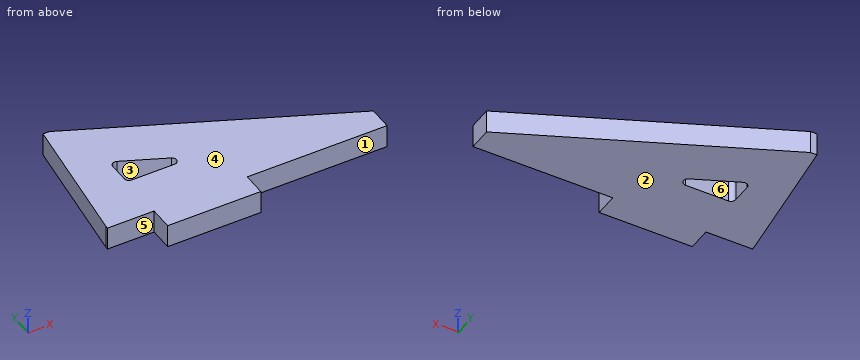
```python
from build123d import *

# Parameters (mm, degrees)
BOSS_EXTRUDE1_DEPTH = 6.35
CUT_EXTRUDE1_DEPTH  = 78.771299333


with BuildPart() as part:
    # Sketch2 → Boss-Extrude1 (new body)
    with BuildSketch(Plane.XY):
        Polygon((0, 0), (0, 6.35), (-12.7, 6.35), (-12.7, 44.45), (-6.35, 44.45), (63.5, 12.7), (63.5, 6.35), (25.4, 6.35), (25.4, 0), align=None)
        with BuildLine():
            Line((0, 25.64089525), (0, 20.32))
            ThreePointArc((0, 20.32), (0.371974388, 19.421974388), (1.27, 19.05))
            Line((1.27, 19.05), (12.97596955, 19.05))
            ThreePointArc((12.97596955, 19.05), (14.217184699, 20.051141386), (13.501499289, 21.476165426))
            Line((13.501499289, 21.476165426), (1.795529739, 26.797060676))
            ThreePointArc((1.795529739, 26.797060676), (0.5824401, 26.708678648), (0, 25.64089525))
        make_face(mode=Mode.SUBTRACT)
    extrude(amount=BOSS_EXTRUDE1_DEPTH)

    # Sketch3 → Cut-Extrude1 (cut, through all)
    with BuildSketch(Plane.XY.offset(6.35)):
        Polygon((-8.09810823, 44.45), (-12.7, 6.970599198), (-12.7, 44.45), align=None)
    extrude(amount=-CUT_EXTRUDE1_DEPTH, mode=Mode.SUBTRACT)


solid = part.part
```
Source: CAD feature listing. Evaluate the final solid. Frame: model axes, mm. Face numbers are marked on the shaded views. A direction names the side the tool comes from. Give positions to 0.01 mm unless a question says otherwise; leave off trailing zeros. Write each loop counter-clockwise with the first axis right and the second up, starting at its lowest first coordinate (ties: lowest second). Pieces come first, ordered by that corner, then holes. Notation, with made-up numbers: (47.25, -39.75) - (84.25, -39.75) arc R28 cw to (84.25, -5.75) - close; hole circle Ø7 at (10.25, 8.5). An arc over 180 degrees is marked (long way). One line per item, written item: value. Start each with the question number.
Q1. Material intervals for probe 1 along X at (y, z) = (7, 2); probe 2 along Y at (x, z) = (7, 1); probe 3 along X at (y, z) = (2, 2.5), sorted ascending. Write a range as from..to.
Q2. First-contact query: pin 1 Ø1.5 at (x, z) = (32, 3) entering from -Y; pin 2 Ø3 at (x, z) = (10, 3) entering from +Y; pin 3 Ø3 at (y, z) = (29, 4.5) entering from -X. Flat tips, straight axial feed; report the tip coordinate or a pass-through.
Q3. Section query C-C, the plane y = 23.5. Return the cut outline in (x, z).
Q4. Set-up query: the marked faces 1, 2 and 3. Return all of +Z, -Z, +X, -X, +Y, -Y with unobstructed straight access to the full face (end or side cutting, diameter ignored); none if empty.
Q5. Section query D-D, the plane x = 50. Return the cut outline in (y, z), then the cut area to 3 significant figures.
Q6. Section query B-B, the plane x = 3. Return the cut outline in (y, z), then the cut area to 3 significant figures.
Q7. Section query A-A, the plane z = 5.5. Return the cut outline in (x, y).
Q8. Draft query along Y for the marked faces 4, 5 and 6. Return one class per face: +Y half, -Y half, draft (parallel to the pull), parting line (faces both ways), or undercut.
Answer:
1. probe 1: x = -12.7..63.5
1. probe 2: y = 0..19.05, 24.43..38.38
1. probe 3: x = 0..25.4
2. pin 1: stops at y = 6.35
2. pin 2: stops at y = 37.7
2. pin 3: stops at x = -10.18
3. outline: (-10.67, 0) - (0, 0) - (0, 6.35) - (-10.67, 6.35) - close; (9.05, 0) - (39.74, 0) - (39.74, 6.35) - (9.05, 6.35) - close
4. face 1: +Z, -Z, +X, -Y
4. face 2: -Z, +X, -X, +Y, -Y
4. face 3: +Z, -Z
5. outline: (6.35, 0) - (18.84, 0) - (18.84, 6.35) - (6.35, 6.35) - close
5. area: 79.3 mm2
6. outline: (0, 0) - (19.05, 0) - (19.05, 6.35) - (0, 6.35) - close; (26.25, 0) - (40.2, 0) - (40.2, 6.35) - (26.25, 6.35) - close
6. area: 210 mm2
7. outline: (-12.7, 6.35) - (0, 6.35) - (0, 0) - (25.4, 0) - (25.4, 6.35) - (63.5, 6.35) - (63.5, 12.7) - (-6.35, 44.45) - (-8.1, 44.45) - (-12.7, 6.97) - close; hole (0, 20.32) arc R1.27 ccw to (1.27, 19.05) - (12.98, 19.05) arc R1.27 ccw to (13.5, 21.48) - (1.8, 26.8) arc R1.27 ccw to (0, 25.64) - close
8. face 4: draft
8. face 5: -Y half
8. face 6: undercut
